from build123d import *

# Parameters (mm, degrees)
ESQUISSE1_R                  = 5
BOSS_EXTRU_1_DEPTH           = 10
ESQUISSE2_R                  = 3
ENL_V_MAT_EXTRU_1_DEPTH      = 10
ENL_V_MAT_EXTRU_2_DEPTH      = 10
ENL_V_MAT_EXTRU_2_DEPTH_BACK = 10
ESQUISSE3_W                  = 6
ESQUISSE3_H                  = 1


with BuildPart() as part:
    # Esquisse1 → Boss.-Extru.1 (new body)
    with BuildSketch(Plane.XY):
        Circle(ESQUISSE1_R)
    extrude(amount=BOSS_EXTRU_1_DEPTH)

    # Esquisse2 → Enlèv. mat.-Extru.1 (cut)
    with BuildSketch(Plane.XY.offset(10)):
        Circle(ESQUISSE2_R)
    extrude(amount=-ENL_V_MAT_EXTRU_1_DEPTH, mode=Mode.SUBTRACT)

    # Esquisse3 → Enlèv. mat.-Extru.2 (cut, two sides: drawn at the far end of the back side and taken through both)
    with BuildSketch(Plane(origin=(0, 0, 0), x_dir=(0, 0, -1), z_dir=(1, 0, 0)).offset(-ENL_V_MAT_EXTRU_2_DEPTH_BACK)):
        with Locations((-3, 4.5)):
            Rectangle(ESQUISSE3_W, ESQUISSE3_H)
        with Locations((-3, -4.5)):
            Rectangle(ESQUISSE3_W, ESQUISSE3_H)
    extrude(amount=ENL_V_MAT_EXTRU_2_DEPTH + ENL_V_MAT_EXTRU_2_DEPTH_BACK, mode=Mode.SUBTRACT)


solid = part.part
Check sheet for the modelled part. Datum: model origin and axes. Units: mm. A direction names the side the tool comes from. Give positions to 0.01 mm unless a question says otherwise; leave off trailing zeros. Loops run counter-clockwise (first coordinate to the right, second up) from the corner with the lowest first, then second, coordinate; pieces in that order, holes last. Notation, with made-up numbers: M 65.25,53.5 L 81.25,53.5 A18 cw 81.25,68.5 Z; hole C -10.5,85 d4. An arc over 180 degrees is marked long. Use a Markdown table: item, result. Add a question column.
Q1. Sectioned sample at B-B, the plane x = 0. Record the cut outline in (y, z), then the cut area to 3 significant figures.
Q2. Tool access check on faces 1 (the flat face through (0, 4, 3)), 2 (the flat face through (0, -4.4, 6)), 3 (the flat face through (3.3, 0.1, 0)). Record the directions out of +Z, -Z, +X, -X, +Y, -Y that give a thin tool (end or side, any length) a straight path to the whole face; none if there is none.
Q3. Go/stop test with flat-tipped pins: pin 1 (0.5 mm diameter, centred on x = -0.5, y = 4.5, fed in from -Z); pin 2 (1.5 mm diameter, centred on x = 0, z = 2.5, fed in from -Y); pin 3 (6 mm diameter, centred on x = 0.5, z = 2.5, fed in from +Y). Record where each tip stops, or that it passes through.
Q4. Sectioned sample at C-C, the plane z = 3.25. Record the cut outline in (x, y), then the cut area to 3 significant figures.
Q5. Sectioned sample at D-D, the plane x = 1.5. Record the cut outline in (y, z).
Q6. Scan lines: line 1 along Y through (x, z) = (0, 7); line 2 along Y through (x, z) = (0, 2.75); line 3 along X through (y, z) = (2.5, 4.25). Record each from-to range of solid material in increasing order. Write a range as [from, to].
Q7. Sectioned sample at A-A, the plane y = 0. Record the cut outline in (x, z).
Q8. Mould release check, pull along X, two halves, no side actions. Record for faces 4 (the cylindrical face through (-3, 0, 5)), 5 (the cylindrical face through (-5, 0, 6)), 6 (the flat face through (-0.1, -3.3, 10)): pulls with the +X half, pulls with the -X half, needs draft (parallel to the pull), parting line crosses it, or undercut.
Verdict:
| question | item | result |
|---|---|---|
| 1 | outline | M -5,6 L -4,6 L -4,0 L -3,0 L -3,10 L -5,10 Z; M 3,0 L 4,0 L 4,6 L 5,6 L 5,10 L 3,10 Z |
| 1 | area | 28.0 mm^2 |
| 2 | face 1 | -Z, +X, -X, +Y |
| 2 | face 2 | -Z, +X, -X, -Y |
| 2 | face 3 | -Z, +X, -X, +Y, -Y |
| 3 | pin 1 | z = 6 |
| 3 | pin 2 | y = -4 |
| 3 | pin 3 | y = 4 |
| 4 | outline | M -3,-4 L 3,-4 A5 ccw 3,4 L -3,4 A5 ccw Z; hole C 0,0 d6 |
| 4 | area | 42.1 mm^2 |
| 5 | outline | M -4.77,6 L -4,6 L -4,0 L -2.6,0 L -2.6,10 L -4.77,10 Z; M 2.6,0 L 4,0 L 4,6 L 4.77,6 L 4.77,10 L 2.6,10 Z |
| 6 | line 1 | [-5, -3], [3, 5] |
| 6 | line 2 | [-4, -3], [3, 4] |
| 6 | line 3 | [-4.33, -1.66], [1.66, 4.33] |
| 7 | outline | M -5,0 L -3,0 L -3,10 L -5,10 Z; M 3,0 L 5,0 L 5,10 L 3,10 Z |
| 8 | face 4 | undercut |
| 8 | face 5 | parting line crosses it |
| 8 | face 6 | needs draft |
